Input: part model. Units: mm. Frame: model coordinates. A direction names the side the tool comes from. Round coordinates to 2 decimals unless told otherwise and drop trailing zeros. Write each loop counter-clockwise with the first axis right and the second up, starting at its lowest first coordinate (ties: lowest second). Pieces come first, ordered by that corner, then holes. Notation, with made-up numbers: (82.5, 3.25) - (122.5, 3.25) arc R24 ccw to (122.5, 23.25) - close; hole circle Ø3 at (60, 46). An arc over 180 degrees is marked (long way). One line per item, written item: value. Start each with the question number.
```python
from build123d import *

# Parameters (mm, degrees)
F0_W     = 65
F0_H     = 150
F1_DEPTH = 3
F2_W     = 55
F2_H     = 3
F3_DEPTH = 3
F4_W     = 3
F4_H     = 15
F5_DEPTH = 3
F6_W     = 3
F6_H     = 75
F7_DEPTH = 40
F8_W     = 15
F8_H     = 3
F9_DEPTH = 3


with BuildPart() as f1:
    # F0 (on Right) → F1 (new body)
    with BuildSketch(Plane.YZ):
        Rectangle(F0_W, F0_H)
    extrude(amount=F1_DEPTH)

    # F2 (on face) → F3 (cut, through all)
    with BuildSketch(Plane.YZ.offset(3)):
        with Locations((5, 73.5)):
            Rectangle(F2_W, F2_H)
    extrude(amount=-F3_DEPTH, mode=Mode.SUBTRACT)

    # F4 (on face) → F5 (cut, through all)
    with BuildSketch(Plane.YZ.offset(3)):
        with Locations((31, 64.5)):
            Rectangle(F4_W, F4_H)
        with Locations((31, 34.5)):
            Rectangle(F4_W, F4_H)
    extrude(amount=-F5_DEPTH, mode=Mode.SUBTRACT)

    # F6 (on face) → F7 (join)
    with BuildSketch(Plane.XZ.offset(32.5)):
        with Locations((1.5, -37.5)):
            Rectangle(F6_W, F6_H)
    extrude(amount=F7_DEPTH)

    # F8 (on face) → F9 (cut, through all)
    with BuildSketch(Plane.YZ.offset(3)):
        with BuildLine():
            Line((-6.735242, 4.372493), (-8.983605, 2.357307))
            ThreePointArc((-8.983605, 2.357307), (13.899524, 2.281442), (16.319635, 25.036362))
            Line((16.319635, 25.036362), (14.071272, 23.021176))
            ThreePointArc((14.071272, 23.021176), (11.897213, 4.51544), (-6.735242, 4.372493))
        make_face()
        with BuildLine():
            ThreePointArc((13.983605, 27.642693), (-8.899524, 27.718558), (-11.319635, 4.963638))
            Line((-11.319635, 4.963638), (-9.071272, 6.978824))
            ThreePointArc((-9.071272, 6.978824), (-6.897213, 25.48456), (11.735242, 25.627507))
            Line((11.735242, 25.627507), (13.983605, 27.642693))
        make_face()
        Polygon((-26.736403, -8.270669), (-32.5, 29.491454), (-32.5, 0), (-72.5, 0), (-72.5, -75), align=None)
        Polygon((-22.420732, -51.427379), (-51.33573, -75), (5.631127, -75), align=None)
        Polygon((8.86788, -31.359509), (32.5, -68.905853), (32.5, -5.897049), align=None)
        with Locations((0, 43.517388)):
            Rectangle(F8_W, F8_H)
    extrude(amount=-F9_DEPTH, mode=Mode.SUBTRACT)


solid = f1.part
```
Q1. Cut plane D-D, the plane y = -48. Output: boundary loops of the cut face in (x, z), and give its area (3 significant figures).
Q2. Cut plane B-B, the plane z = -55. Output: boundary loops of the cut face in (x, y), and give its area (3 significant figures).
Q3. Material intervals for probe 1 along Y at (x, z) = (0.35, 28); probe 2 along Z at (x, y) = (2.8, 5); probe 3 along Z at (x, y) = (0.85, 0), sorted ascending. Write a range as from..to.
Q4. Cut plane C-C, the plane y = 2. Output: boundary loops of the cut face in (x, z), and give its area (3 significant figures).
Q5. Contact query for flat-ended pins moving along their axis: pin 1 Ø1.5 at (x, y) = (1.5, 30.5) entering from +Z; pin 2 Ø1.5 at (x, z) = (1.5, 33.5) entering from +Y. Output: stop coordinate, or through.
Q6. Access query for faces 4 (the flat face through (2, 3, 72)), 5 (the flat face through (1, -32.5, 52)), 6 (the flat face through (1.52, -36.68, -63.05)). Directions: +Z, -Z, +X, -X, +Y, -Y. A direction counts if a zero-diameter tool reaches every point of the face in a straight line with its end or side. Return the directions, or none.
Q7. Cut plane A-A, the plane x = 2. Count the separate pieces of the cut face and the enclosed holes in it, and give its area (3 significant figures).
Q8. Pull-direction query (Y, two-part tool) for faces 1 (the cylindrical face through (1.5, -7.1, 25.3)), 2 (the flat face through (1, 32.5, 10)), 3 (the flat face through (1, -62, -75)); classes: pulls with the +Y half, pulls with the -Y half, needs draft (parallel to the pull), parting line crosses it, or undercut.
A:
1. outline: (0, -72.28) - (3, -72.28) - (3, -39.28) - (0, -39.28) - close
1. area: 99.0 mm²
2. outline: (0, -58.78) - (3, -58.78) - (3, -26.8) - (0, -26.8) - close; (0, -18.17) - (3, -18.17) - (3, 23.75) - (0, 23.75) - close
2. area: 222 mm²
3. probe 1: y = -32.27..-8.58, -2.91..7.91, 13.58..29.5
3. probe 2: z = -74.47..-1.9, 1.14..28.86, 31.9..42.02, 45.02..72
3. probe 3: z = -70.27..-1.9, 1.14..28.86, 31.9..42.02, 45.02..72
4. outline: (0, -71.95) - (3, -71.95) - (3, -2.07) - (0, -2.07) - close; (0, 0.93) - (3, 0.93) - (3, 29.07) - (0, 29.07) - close; (0, 32.07) - (3, 32.07) - (3, 42.02) - (0, 42.02) - close; (0, 45.02) - (3, 45.02) - (3, 72) - (0, 72) - close
4. area: 405 mm²
5. pin 1: stops at z = 57
5. pin 2: stops at y = 29.5
6. face 4: +Z, +X, -X, +Y
6. face 5: +Z, +X, -X, -Y
6. face 6: -Z, +X, -X
7. separate pieces: 1
7. enclosed holes: 3
7. area: 8,790 mm²
8. face 1: undercut
8. face 2: pulls with the +Y half
8. face 3: needs draft
